Geometry: see drawing. Coordinates: mm, zero at the bounding-box minimum. Give positions to 0.01 mm unless a question says otherwise; leave off trailing zeros. Write each loop counter-clockwise with the first axis right and the second up, starting at its lowest first coordinate (ties: lowest second). Pieces come first, ordered by that corner, then holes. Notation, with made-up numbers: M 1.25,21.5 L 40.25,21.5 A21 cw 40.25,28.5 Z; hole C -22,58.5 d8. An arc over 180 degrees is marked long. Use a Markdown table: item, result. Add a question column.
1) Pin query (flat end, axial travel): pin 1 (0.9 mm diameter, centred on x = 1.5, z = 1.5, fed in from -Y); pin 2 (4 mm diameter, centred on x = 55.5, y = 30.5, fed in from -Z); pin 3 (1 mm diameter, centred on y = 6, z = 2, fed in from -X). Return the tip coordinate at first contact, or that it passes through.
2) Line query: line 1 (Y direction, x = 4, z = 2.2); line 2 (X direction, y = 32, z = 0.65); line 3 (X direction, y = 2, z = 0.6). Output: solid intervals per line, ascending.
3) Section A-A on z = 1.4. Return the cut outline in (x, y), then the cut area to 4 significant figures.
4) Section C-C on y = 19.5. Return the cut outline in (x, z), then the cut area to 3 significant figures.
5) Section B-B on x = 43.5. Return the cut outline in (y, z), then the cut area to 4 significant figures.
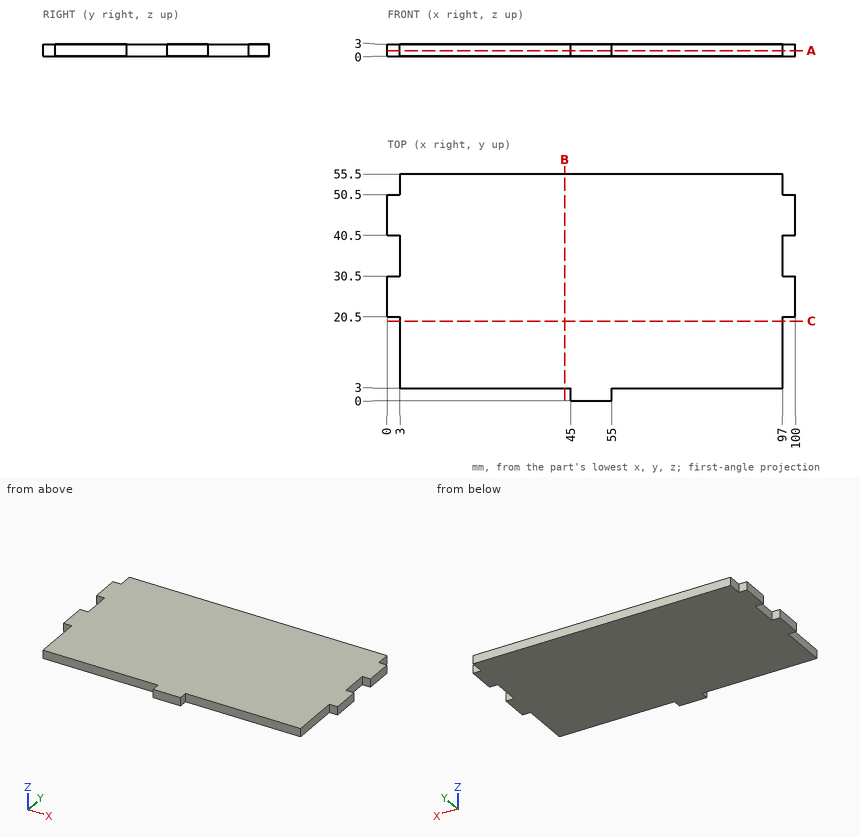
Found:
| question | item | result |
|---|---|---|
| 1 | pin 1 | y = 20.5 |
| 1 | pin 2 | z = 0 |
| 1 | pin 3 | x = 3 |
| 2 | line 1 | 3 to 55.5 |
| 2 | line 2 | 3 to 97 |
| 2 | line 3 | 45 to 55 |
| 3 | outline | M 0,20.5 L 3,20.5 L 3,3 L 45,3 L 45,0 L 55,0 L 55,3 L 97,3 L 97,20.5 L 100,20.5 L 100,30.5 L 97,30.5 L 97,40.5 L 100,40.5 L 100,50.5 L 97,50.5 L 97,55.5 L 3,55.5 L 3,50.5 L 0,50.5 L 0,40.5 L 3,40.5 L 3,30.5 L 0,30.5 Z |
| 3 | area | 5,085 mm² |
| 4 | outline | M 3,0 L 97,0 L 97,3 L 3,3 Z |
| 4 | area | 282 mm² |
| 5 | outline | M 3,0 L 55.5,0 L 55.5,3 L 3,3 Z |
| 5 | area | 157.5 mm² |
